CAD build for the part. Positions are in the model's coordinates, mm. Round coordinates to 2 decimals unless told otherwise and drop trailing zeros. Write each loop counter-clockwise with the first axis right and the second up, starting at its lowest first coordinate (ties: lowest second). Pieces come first, ordered by that corner, then holes. Notation, with made-up numbers: (23, 62) - (52, 62) arc R7 ccw to (52, 66) - close; hole circle Ø5 at (6, 38). An arc over 180 degrees is marked (long way). Put each result on its own line as item: value. Start each with the question number.
Item 1: Cut at D-D (z = 11.25). Give the cut face in (x, y), and give its area (3 significant figures).
Item 2: Cut at C-C (z = 1.5). Give the cut face in (x, y), and give its area (3 significant figures).
Item 3: Cut at A-A (x = 50.5). Give the cut face in (y, z).
Item 4: Pin check, flat tips, straight feed: pin 1 Ø0.9 at (y, z) = (18, 2) entering from +X; pin 2 Ø10 at (y, z) = (-12.5, 20) entering from +X; pin 3 Ø0.9 at (y, z) = (16.5, 2) entering from -X. Stop position of each tip, or through.
Item 5: Drill centre lines: line 1 (X direction, y = 48.5, z = 1.75); line 2 (Y direction, x = -20, z = 21.75). Where is each one in solid material? Low to high. Write a range as from..to.
Item 6: Cut at B-B (y = 37.5). Give the cut face in (x, z), and give its area (3 significant figures).
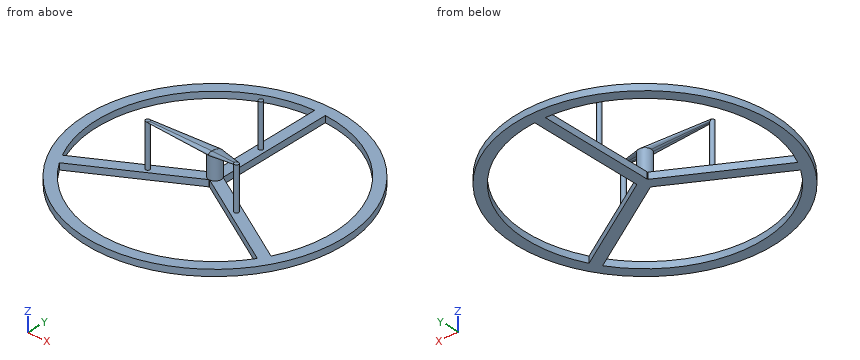
Autodesk Fusion 360 part; units mm, degrees
sketch "スケッチ1" plane through (0, 0, 0) normal (0, 0, 1) x (1, 0, 0)
  circle A0 centre (0, 0) radius 76
  line L0 (-25, 0) -> (125, 0)
  circle A1 centre (120, 0) radius 5
  ellipse E0 centre (0, 0) end of major axis (125, 0) minor radius 90
  line L1 (-125, 0) -> (125, 0)
  line L2 (0, -90) -> (0, 90)
  ellipse E1 centre (0, 0) end of major axis (115, 0) minor radius 80
  line L3 (-115, 0) -> (115, 0)
  line L4 (0, -80) -> (0, 80)
  circle A2 centre (0, 85) radius 5
  circle A3 centre (0, -85) radius 5
  line L5 (120, 0) -> (115, 0)
  line L6 (120, 5) -> (120, 0)
  line L7 (115, 5) -> (125, 5)
  line L8 (125, 5) -> (125, -5)
  line L9 (125, -5) -> (115, -5)
  line L10 (115, -5) -> (115, 5)
  dimension "d1" = 152
  dimension "d2" = 150
extrude "押し出し1" add sketch "スケッチ1" along normal blind 141 contours A0 L0 L1 L2 L3 L4 | A0 L0 L1 L2 L3 L4 | A0 L0 L1 L2 L3 L4 | A0 L0 L1 L2 L3 L4 makes body 1
extrude "押し出し2" add sketch "スケッチ1" along normal blind 3 separate body contours E0 E1 A3 L9 L10 | E0 E1 A2 L7 L10 | L2 A2 | L2 A2 | L2 A3 | L2 A3 makes body 2 at (30.5782, -83.5354, 0)
sketch "スケッチ2" plane through (0, 0, 0) normal (0, 1, 0) x (1, 0, 0)
  line L0 (0, -170) -> (100, -170)
  line L1 (120, -150) -> (120, 0)
  arc A0 (100, -170) -> (120, -150) centre (100, -150) ccw
  line L2 (0, -170) -> (0, -175)
  line L3 (0, -175) -> (100, -175)
  line L4 (100, -175) -> (100, -165)
  line L5 (100, -165) -> (0, -165)
  line L6 (0, -165) -> (0, -175)
  circle A1 centre (100, -150) radius 15
  circle A2 centre (100, -150) radius 25
  line L7 (125, -150) -> (115, -150)
  line L8 (115, -150) -> (115, 0)
  line L9 (115, 0) -> (125, 0)
  line L10 (125, 0) -> (125, -150)
  dimension "d11" = 20
  dimension "d24" = 5
  dimension "d25" = 100
  dimension "d26" = 10
ref_plane "作業平面1" through (0, 0, 170) normal (0, 0, 1) x (1, 0, 0)
sketch "スケッチ3" plane through (0, 0, 170) normal (0, 0, 1) x (1, 0, 0)
  circle A0 centre (0, 0) radius 3
  circle A1 centre (0, 0) radius 5
  circle A2 centre (0, 0) radius 2.5
  line L0 (0, 0) -> (-5, 0)
  line L1 (0, 0) -> (-2.5, 4.3301)
  line L2 (0, 0) -> (-2.5, -4.3301)
  circle A3 centre (-1.875, 3.2476) radius 1.25
  circle A4 centre (-1.875, -3.2476) radius 1.25
  line L3 (0, 0) -> (5, 0)
  line L4 (0, 0) -> (0, 5)
  line L5 (0, 0) -> (0, -5)
  arc A5 (0, 3) -> (-1.25, 2.1651) centre (-0.2231, 1.9809) ccw
  arc A6 (-1.25, -2.1651) -> (0, -3) centre (-0.2231, -1.9809) ccw
  dimension "d17" = 6
  dimension "d18" = 10
  dimension "d23" = 5
extrude "押し出し4" add sketch "スケッチ3" along normal mid plane 10 separate body contours A0 A1 L3 L5 | A0 A1 L3 L4 | A1 A3 L4 A5 | A0 A5 | A0 A6 | A1 A4 L5 A6 | A0 L1 A5 | A0 L1 A3 | A0 L2 A4 | A0 L2 A6 | A0 L1 A3 | A0 L1 A3 | A0 L2 A4 | A0 L2 A4 makes body 3
extrude "押し出し6" add sketch "スケッチ2" along normal mid plane 10 contours L0 L5 L6 A2 | L0 L2 L3 L6 A2 | L0 L4 L5 A2 | L0 L4 A2 | A0 L4 A1 L7 | A0 L4 A2 L7 | L1 A2 L7 L8 | L1 A2 L7 | L1 A2 L8 L9 | L1 A2 L9 L10 bodies 3 2
extrude "押し出し5" cut sketch "スケッチ3" along normal mid plane 10 contours A0 A2 L3 L4 | A0 A2 L3 L5 | A0 A2 A3 L4 | A0 A6 | A0 A2 A4 L5 | A2 L3 L4 | A2 L3 L5 | A3 A5 | A2 L1 L4 | A4 A6 bodies 3
extrude "押し出し7" cut sketch "スケッチ1" along normal blind 175 contours E0 L8 L9 | E0 L7 L8 bodies 3
sketch "スケッチ4" plane through (0, 0, 0) normal (0, 0, 1) x (1, 0, 0)
  circle A0 centre (85, 0) radius 3
  circle A1 centre (75, 0) radius 3
  dimension "d66" = 6
  dimension "d68" = 6
extrude "押し出し8" add sketch "スケッチ4" along normal blind 150 separate body makes body 4 at (85.8125, 2.8879, 100) makes body 5 at (75.8125, 2.8879, 100)
sketch "スケッチ5" plane through (0, 0, 150) normal (0, 0, 1) x (-1, 0, 0)
  circle A0 centre (-85, 0) radius 3
  circle A1 centre (-75, 0) radius 3
  circle A2 centre (-85, 0) radius 1.5
  circle A3 centre (-75, 0) radius 1.6
  dimension "d69" = 3
  dimension "d70" = 3.2
extrude "押し出し9" add sketch "スケッチ5" along normal blind 3 contours A2 bodies 4
extrude "押し出し10" cut sketch "スケッチ5" against normal blind 3 contours A3 bodies 5
sketch "スケッチ6" plane through (0, 0, 0) normal (0, 0, 1) x (1, 0, 0)
  circle A0 centre (0, 0) radius 60
  circle A1 centre (0, 0) radius 55
  circle A2 centre (0, 0) radius 25
  line L0 (0, 0) -> (0, 60)
  line L1 (2.5, 55) -> (2.5, 0)
  line L2 (2.5, 0) -> (-2.5, 0)
  line L3 (-2.5, 0) -> (-2.5, 55)
  line L4 (1.25, -2.1651) -> (-46.3814, -29.6651)
  line L5 (-48.8814, -25.3349) -> (-1.25, 2.1651)
  line L6 (-1.25, 2.1651) -> (1.25, -2.1651)
  line L7 (1.25, 2.1651) -> (48.8814, -25.3349)
  line L8 (46.3814, -29.6651) -> (-1.25, -2.1651)
  line L9 (-1.25, -2.1651) -> (1.25, 2.1651)
  circle A3 centre (0, 0) radius 3
  dimension "d41" = 50
  dimension "d43" = 5
  dimension "d45" = 360
  dimension "d48" = 6
extrude "押し出し11" add sketch "スケッチ6" along normal blind 3 separate body contours A1 A2 L0 L1 | A1 A2 L0 L3 | A0 | A2 L0 L3 A3 | A2 L0 L1 A3 | A1 A2 L4 L5 | L0 L1 L7 L9 A3 | L0 L3 L5 L6 A3 | A1 A2 L7 L8 | A2 L4 L5 A3 | L1 L2 L7 L9 | L2 L3 L4 L5 L8 L9 A3 | L2 L3 L5 L6 | L1 L2 L4 L6 L7 L8 A3 | L4 L6 L8 L9 | A2 L7 L8 A3 makes body 6
extrude "押し出し12" add sketch "スケッチ6" along normal blind 13 contours L0 L1 L7 L9 A3 | L0 L3 L5 L6 A3 | L1 L7 A3 | L3 L5 A3 | L1 L2 L7 L9 | L2 L3 L4 L5 L8 L9 A3 | L2 L3 L5 L6 | L1 L2 L4 L6 L7 L8 A3 | L4 L6 L8 L9 | L4 L8 A3 bodies 6
ref_plane "作業平面2" through (0, 0, 23) normal (0, 0, 1) x (1, 0, 0)
sketch "スケッチ7" plane through (0, 0.0029, 23) normal (0, 0, 1) x (1, 0, 0)
  circle A0 centre (0, 0) radius 25
  line L0 (0, 0) -> (25, 0) construction
  line L1 (0, 0) -> (26.2494, 0) construction
  line L2 (0, 0) -> (28.4476, 0) construction
  circle A1 centre (-20.7846, -12) radius 1
  circle A2 centre (20.7846, -12) radius 1
  circle A3 centre (0, 24) radius 1
  dimension "d61" = 2
  dimension "d62" = 2
  dimension "d63" = 2
sketch "スケッチ8" plane through (0, 0, 13) normal (0, 0, 1) x (-1, 0, 0)
  circle A0 centre (0, 0) radius 3
  circle A1 centre (0, 0) radius 3
loft "ロフト1" add profiles "スケッチ8", "スケッチ7" section 1 section 2 contours A3 bodies 6
loft "ロフト2" add profiles "スケッチ8", "スケッチ7" section 1 section 2 contours A1 bodies 6
loft "ロフト3" add profiles "スケッチ8", "スケッチ7" section 1 section 2 contours A2 bodies 6
extrude "押し出し13" add sketch "スケッチ7" against normal blind 20 contours A3 | A1 | A2 bodies 6
hidden bodies 1 3 4 5
Output values:
1. outline: circle Ø2 at (-20.78, -12); circle Ø6 at (0, 0); circle Ø2 at (0, 24); circle Ø2 at (20.78, -12)
1. area: 37.7 mm2
2. outline: circle Ø120 at (0, 0); hole (-48.83, -25.31) - (-2.69, 1.34) arc R3 cw to (-2.5, 1.66) - (-2.5, 54.94) arc R55 ccw to start; hole (-46.33, -29.64) arc R55 ccw to (46.33, -29.64) - (0.19, -2.99) arc R3 cw to (-0.19, -2.99) - close; hole (2.5, 1.66) arc R3 cw to (2.69, 1.34) - (48.83, -25.31) arc R55 ccw to (2.5, 54.94) - close
2. area: 2,620 mm2
3. outline: (-32.4, 0) - (-21.79, 0) - (-21.79, 3) - (-32.4, 3) - close; (21.79, 0) - (32.4, 0) - (32.4, 3) - (21.79, 3) - close
4. pin 1: x = 57.38
4. pin 2: x = 21.78
4. pin 3: x = -57.81
5. line 1: -35.32..-25.94, -2.5..2.5, 25.94..35.32
5. line 2: -12.62..-11.38
6. outline: (-46.84, 0) - (-40.23, 0) - (-40.23, 3) - (-46.84, 3) - close; (-2.5, 0) - (2.5, 0) - (2.5, 3) - (-2.5, 3) - close; (40.23, 0) - (46.84, 0) - (46.84, 3) - (40.23, 3) - close
6. area: 54.6 mm2
